Verification items for this drawing (mm, ordinates from the low corner). A direction names the side the tool comes from. Coordinates: 2 decimals unless noted, no trailing zeros. Order: outer loops, then holes, each group sorted by start corner. A loop starts at its lowest first (then second) coordinate and runs counter-clockwise, first axis right, second up. Notation, with made-up numbers: (44, 84.5) -> (75, 84.5) arc R14 cw to (75, 106.5) -> close; hole circle Ø3 at (24.5, 72). An arc over 180 degrees is marked (long way). Answer in a Markdown table with one row per item. Add a question column.
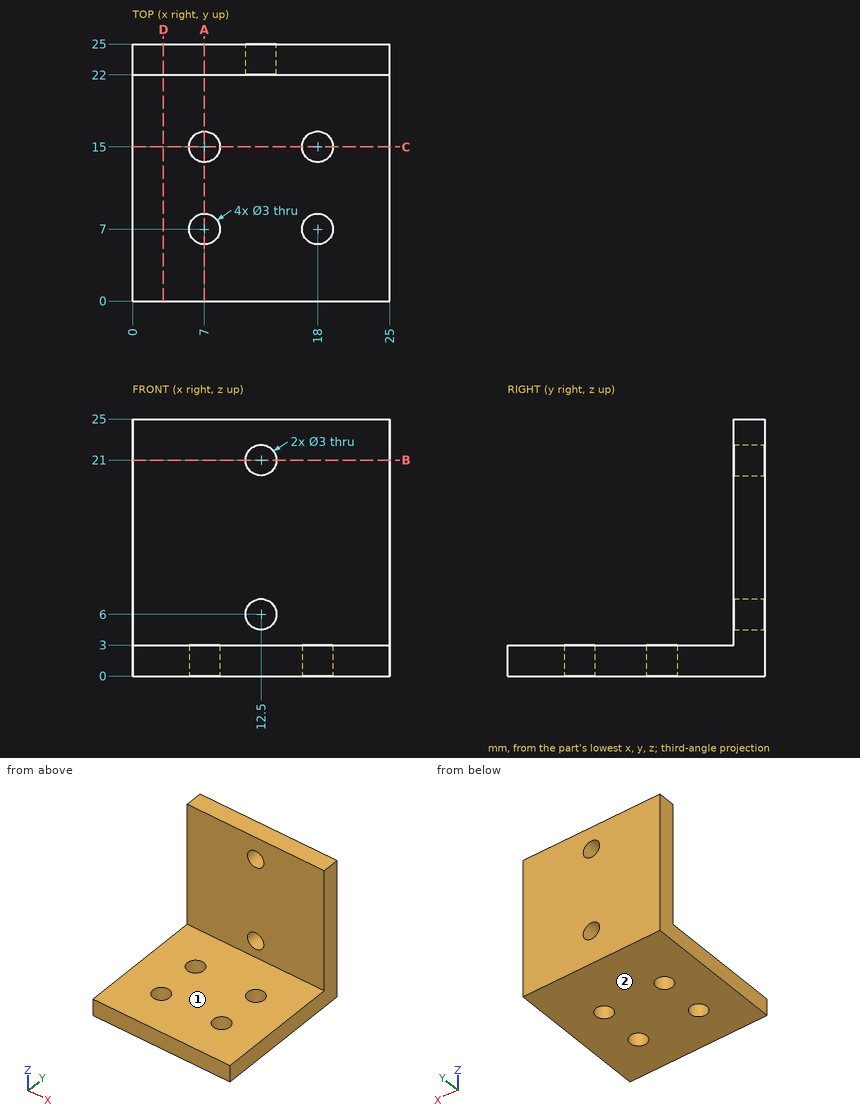
(1) Scan lines: line 1 along Z through (x, y) = (12.5, 24.25); line 2 along X through (y, z) = (16.25, 1.5); line 3 along Y through (x, z) = (17.5, 15.25). Record each from-to range of solid material in increasing order.
(2) Go/stop test with flat-tipped pins: P1, Ø3.5, axis at x = 12.5, z = 21, coming from the -Y side; P2, Ø6.5, axis at x = 17.5, y = 8.5, coming from the +Z side; P3, Ø1.8, axis at x = 7, y = 15, coming from the +Z side. Record where each tip stops, or that it passes through.
(3) Cross-section at D-D (x = 3). Enter the section's corners in (y, z).
(4) Cross-section at C-C (y = 15). Enter the section's corners in (x, z), plus the area to 3 significant figures.
(5) Cross-section at B-B (z = 21). Enter the section's corners in (x, y), plus the area to 3 significant figures.
(6) Access from +Z, -Z, +X, -X, +Y, -Y to the whole of each face (thin tool, end or side, straight path). Record for the marked faces 1 and 2.
(7) Cross-section at A-A (x = 7). Enter the section's corners in (y, z), plus the area to 3 significant figures.
Checks:
| question | item | result |
|---|---|---|
| 1 | line 1 | 0 to 4.5, 7.5 to 19.5, 22.5 to 25 |
| 1 | line 2 | 0 to 6.17, 7.83 to 17.17, 18.83 to 25 |
| 1 | line 3 | 22 to 25 |
| 2 | P1 | y = 22 |
| 2 | P2 | z = 3 |
| 2 | P3 | through |
| 3 | outline | (0, 0) -> (25, 0) -> (25, 25) -> (22, 25) -> (22, 3) -> (0, 3) -> close |
| 4 | outline | (0, 0) -> (5.5, 0) -> (5.5, 3) -> (0, 3) -> close; (8.5, 0) -> (16.5, 0) -> (16.5, 3) -> (8.5, 3) -> close; (19.5, 0) -> (25, 0) -> (25, 3) -> (19.5, 3) -> close |
| 4 | area | 57.0 mm² |
| 5 | outline | (0, 22) -> (11, 22) -> (11, 25) -> (0, 25) -> close; (14, 22) -> (25, 22) -> (25, 25) -> (14, 25) -> close |
| 5 | area | 66.0 mm² |
| 6 | face 1 | +Z, +X, -X, -Y |
| 6 | face 2 | -Z, +X, -X, +Y, -Y |
| 7 | outline | (0, 0) -> (5.5, 0) -> (5.5, 3) -> (0, 3) -> close; (8.5, 0) -> (13.5, 0) -> (13.5, 3) -> (8.5, 3) -> close; (16.5, 0) -> (25, 0) -> (25, 25) -> (22, 25) -> (22, 3) -> (16.5, 3) -> close |
| 7 | area | 123 mm² |
